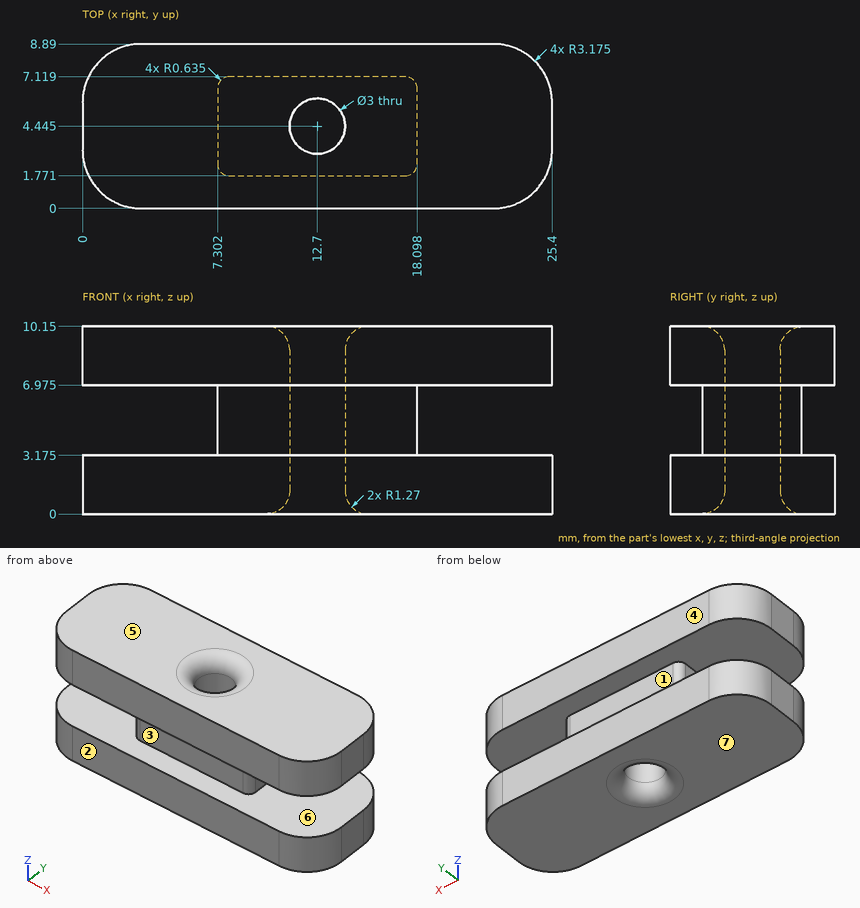
Geometry: see drawing. Coordinates: mm, zero at the bounding-box minimum. A direction names the side the tool comes from. Give positions to 0.01 mm unless a question says otherwise; leave off trailing zeros.
Q1. Draft query along Z for the marked faces 4, 5, 6 and 7. Return one class per face: +Z half, -Z half, draft (parallel to the pull), parting line (faces both ways), or undercut.
Checked values:
face 4: draft
face 5: +Z half
face 6: undercut
face 7: -Z half
Q2. Contact query for flat-ended pins moving along their axis: pin 1 Ø3.5 at (x, y) = (12.7, 4.445) entering from +Z (1 decimal); pin 2 Ø3 at (y, z) = (4.5, 5) entering from +X; pin 3 Ø1.9 at (y, z) = (3.5, 4.5) entering from -X. Output: stop coordinate, or through.
Checked values:
pin 1: stops at z = 9.6
pin 2: stops at x = 18.1
pin 3: stops at x = 7.3
Q3. Ray query, probe 1 along Y at (x, z) = (12.7, 3.25) (1 decimal); probe 2 along Y at (x, z) = (12.7, 7.25) (1 decimal); probe 3 along X at (y, z) = (4, 9). Return the intervals inside material, ascending.
Checked values:
probe 1: y = 1.8 to 2.9, 5.9 to 7.1
probe 2: y = 0 to 2.9, 5.9 to 8.9
probe 3: x = 0 to 11.26, 14.14 to 25.4
Q4. Set-up query: the marked faces 1, 2 and 3. Return all of +Z, -Z, +X, -X, +Y, -Y with unobstructed straight access to the full face (end or side cutting, diameter ignored); none if empty.
Checked values:
face 1: +X, -X, +Y
face 2: +Z, -Z, +X, -X, -Y
face 3: +X, -X, -Y
